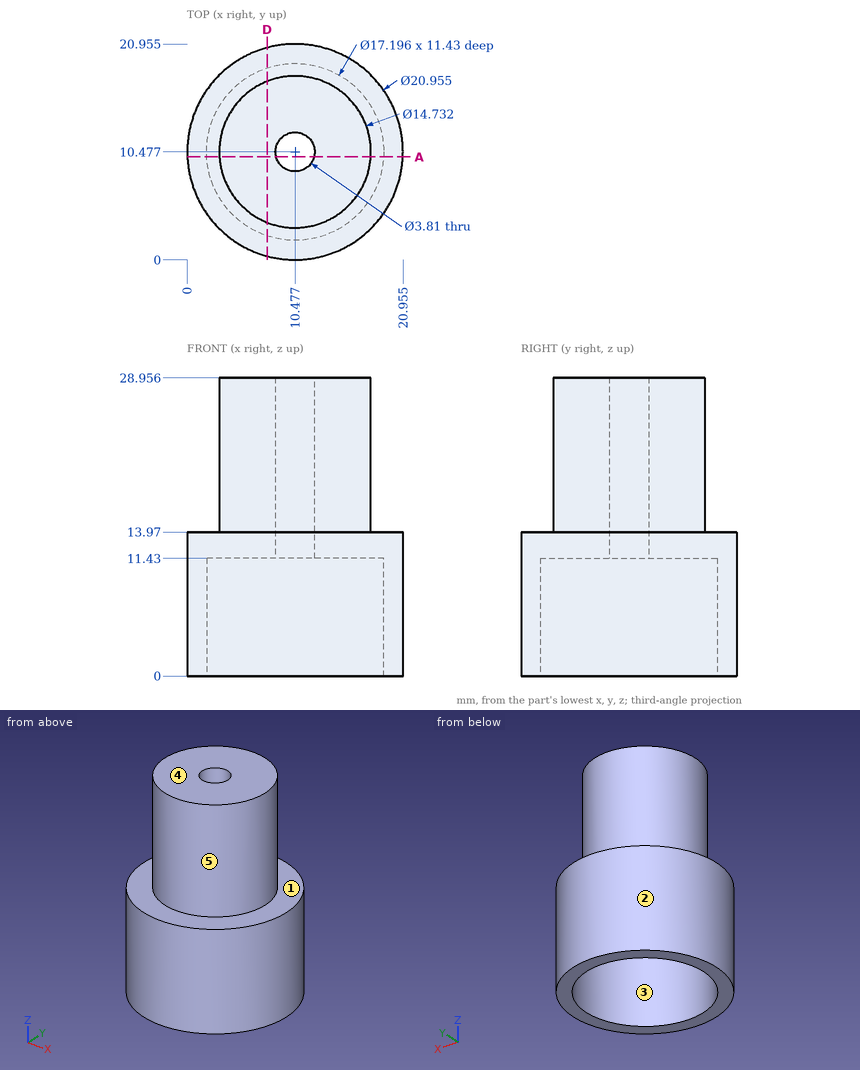
Part print with two shaded views. Sizes in mm from the minimum x, y, z corner. A direction names the side the tool comes from. Coordinates: 2 decimals unless noted, no trailing zeros. Order: outer loops, then holes, each group sorted by start corner. A loop starts at its lowest first (then second) coordinate and runs counter-clockwise, first axis right, second up. Notation, with made-up numbers: M -14.75,53 L 38.25,53 A13 cw 38.25,70 Z; hole C -37,40 d10. An arc over 180 degrees is marked long. Use a Markdown table: item, result.
(1) Probe L1, parallel to Y at x = 10.5, z = 15.5; L2, parallel to Z at x = 8.5, y = 4.5 (1 decimal); L3, parallel to Y at x = 10.75, z = 3. List the from-to ranges inside material, lowest first.
A:
| item | result |
|---|---|
| L1 | y = 3.11 to 8.57, 12.38 to 17.84 |
| L2 | z = 11.4 to 29 |
| L3 | y = 0 to 1.88, 19.07 to 20.95 |
(2) Flat gauge pins, fed straight in: pin 1 (3 mm diameter, centred on x = 10.5, z = 26, fed in from -Y); pin 2 (6 mm diameter, centred on x = 3, z = 11, fed in from +Y); pin 3 (1.5 mm diameter, centred on y = 9.5, z = 10.5, fed in from +X). Where does each tip first touch, or does it go through?
A:
| item | result |
|---|---|
| pin 1 | stops at y = 3.11 |
| pin 2 | stops at y = 19.95 |
| pin 3 | stops at x = 20.95 |
(3) Tool access for the marked faces 1 and 2: list every direction of +Z, -Z, +X, -X, +Y, -Y with a clear straight run to the whole face (end or side of a thin tool).
A:
| item | result |
|---|---|
| face 1 | +Z |
| face 2 | +Z, -Z |
(4) Pull direction X, two halves, no side cores. Call the marked faces 3, 4 and 5: released by +X, released by -X, zero draft, split by the parting line, or undercut.
A:
| item | result |
|---|---|
| face 3 | undercut |
| face 4 | zero draft |
| face 5 | split by the parting line |
(5) Cut at D-D on x = 7.75. Write the cut outline in (y, z) (1 decimal).
A:
| item | result |
|---|---|
| outline | M 0.4,0 L 2.3,0 L 2.3,11.4 L 18.6,11.4 L 18.6,0 L 20.6,0 L 20.6,14 L 17.3,14 L 17.3,29 L 3.6,29 L 3.6,14 L 0.4,14 Z |
(6) Cut at A-A on y = 10. Write the cut outline in (x, z) (1 decimal).
A:
| item | result |
|---|---|
| outline | M 0,0 L 1.9,0 L 1.9,11.4 L 8.6,11.4 L 8.6,29 L 3.1,29 L 3.1,14 L 0,14 Z; M 12.3,11.4 L 19.1,11.4 L 19.1,0 L 20.9,0 L 20.9,14 L 17.8,14 L 17.8,29 L 12.3,29 Z |
